Input: part model. Units: mm. Frame: model coordinates. A direction names the side the tool comes from. Give positions to 0.01 mm unless a question says otherwise; leave off trailing zeros. Order: outer loops, then holes, each group sorted by start corner. A loop starts at its lowest first (then second) coordinate and runs counter-clockwise, first axis right, second up. Notation, with made-up numbers: (68.25, 48.25) - (125.25, 48.25) arc R18 cw to (125.25, 67.25) - close; hole circle Ø2 at (-38.5, 8.25). An arc over 180 degrees is marked (long way). Answer in a Markdown table with one row per item. Add a question column.
1. Contact query for flat-ended pins moving along their axis: pin 1 (1.5 mm diameter, centred on y = 31.5, z = 6.5, fed in from +X); pin 2 (0.7 mm diameter, centred on y = 34.5, z = 516, fed in from +X); pin 3 (5 mm diameter, centred on x = -1, z = 219.5, fed in from +Y). Output: stop coordinate, or through.
2. Ray query, line 1 (Z direction, x = 4.5, y = 17.5); line 2 (Z direction, x = -6.5, y = 12); line 3 (Y direction, x = 6.25, z = 305). Return the intervals inside material, ascending. Write a range as [from, to].
3. Section query A-A on z = 353.5. Return loops of the section in (x, y), and give its area (3 significant figures).
4. Access query for faces 5 (the face through (-1, 15, 11)), 6 (the face through (7.5, 15.6, 521.3)), 7 (the face through (11.9, 16, 2)). Directions: +Z, -Z, +X, -X, +Y, -Y. A direction counts if a zero-diameter tool reaches every point of the face in a straight line with its end or side. Return the directions, or none.
5. Mould query, pull axis X, two halves, no side actions, for faces 1 (the face through (5, 34.5, 259)), 2 (the face through (-1, 16, 5)), 3 (the face through (-12.5, 15, 259)), 4 (the face through (7.5, 15.6, 4.7)). Classes: released by +X, released by -X, zero draft, split by the parting line, or undercut.
```python
from build123d import *

# Parameters (mm, degrees)
EXTRUDE_1_DEPTH          = 526
SKETCH_2_W               = 10
SKETCH_2_H               = 0.6
CUT_EXTRUDE_1_DEPTH      = 14.5
EXTRUDE_START            = -12.5
EXTRUDE_2_DEPTH          = 5
CUT_EXTRUDE_2_DEPTH      = 4.4
CUT_EXTRUDE_3_DEPTH      = 26
CUT_EXTRUDE_4_DEPTH      = 5.5
CUT_EXTRUDE_4_DEPTH_BACK = 5.5
CUT_EXTRUDE_5_DEPTH      = 35.5
SKETCH_8_W               = 0.5
SKETCH_8_H               = 1
CUT_EXTRUDE_8_DEPTH      = 491


with BuildPart() as part:
    # Эскиз1 → Бобышка-Вытянуть1 (new body)
    with BuildSketch(Plane.XY):
        with BuildLine():
            Line((-11.8, 32.5), (-11.8, 28.3))
            Line((-11.8, 28.3), (-11, 27.5))
            Line((-11, 27.5), (-11, 26))
            Line((-11, 26), (-12.5, 24.5))
            Line((-12.5, 24.5), (-12.5, 5))
            ThreePointArc((-12.5, 5), (-11.035533906, 1.464466094), (-7.5, 0))
            Line((-7.5, 0), (7.5, 0))
            ThreePointArc((7.5, 0), (11.035533906, 1.464466094), (12.5, 5))
            Line((12.5, 5), (12.5, 26.5))
            Line((12.5, 26.5), (11.7, 27.3))
            Line((11.7, 27.3), (11.7, 28.5))
            Line((11.7, 28.5), (12.5, 29.3))
            Line((12.5, 29.3), (12.5, 32.5))
            ThreePointArc((12.5, 32.5), (11.914213562, 33.914213562), (10.5, 34.5))
            Line((10.5, 34.5), (-9.8, 34.5))
            ThreePointArc((-9.8, 34.5), (-11.214213562, 33.914213562), (-11.8, 32.5))
        make_face()
    extrude(amount=EXTRUDE_1_DEPTH)

    # Эскиз2 → Вырез-Вытянуть1 (cut)
    with BuildSketch(Plane(origin=(0, 0, 0), x_dir=(-1, 0, 0), z_dir=(0, 0, -1))):
        with BuildLine():
            ThreePointArc((-10.5, 33.9), (-11.489949494, 33.489949494), (-11.9, 32.5))
            Line((-11.9, 32.5), (-11.9, 29.548528137))
            Line((-11.9, 29.548528137), (-11.1, 28.748528137))
            Line((-11.1, 28.748528137), (-11.1, 27.051471863))
            Line((-11.1, 27.051471863), (-11.9, 26.251471863))
            Line((-11.9, 26.251471863), (-11.9, 5))
            ThreePointArc((-11.9, 5), (-10.611269837, 1.888730163), (-7.5, 0.6))
            Line((-7.5, 0.6), (-7.5, 0))
            ThreePointArc((-7.5, 0), (-11.035533906, 1.464466094), (-12.5, 5))
            Line((-12.5, 5), (-12.5, 26.5))
            Line((-12.5, 26.5), (-11.7, 27.3))
            Line((-11.7, 27.3), (-11.7, 28.5))
            Line((-11.7, 28.5), (-12.5, 29.3))
            Line((-12.5, 29.3), (-12.5, 32.5))
            ThreePointArc((-12.5, 32.5), (-11.914213562, 33.914213562), (-10.5, 34.5))
            Line((-10.5, 34.5), (-10.5, 33.9))
        make_face()
        with Locations((0, 0.3)):
            Rectangle(SKETCH_2_W, SKETCH_2_H)
    cut_extrude_1 = extrude(amount=-CUT_EXTRUDE_1_DEPTH, mode=Mode.SUBTRACT)

    # Эскиз5 → Бобышка-Вытянуть2 (add)
    with BuildSketch(Plane.XY.offset(526).offset(EXTRUDE_START)):
        Polygon((-4.5, 34.5), (-2.7, 36.3), (2.7, 36.3), (4.5, 34.5), align=None)
    extrude_2 = extrude(amount=-EXTRUDE_2_DEPTH)

    # Зеркальное отражение1: Вырез-Вытянуть1, Бобышка-Вытянуть2 across plane
    add(cut_extrude_1.mirror(Plane.XY.offset(263)), mode=Mode.SUBTRACT)
    add(extrude_2.mirror(Plane.XY.offset(263)))

    # Эскиз3 → Вырез-Вытянуть2 (cut)
    with BuildSketch(Plane(origin=(11.9, 0, 0), x_dir=(0, 0, -1), z_dir=(1, 0, 0))):
        with BuildLine():
            Line((-523, 14), (-523, 17))
            ThreePointArc((-523, 17), (-518, 22), (-513, 17))
            Line((-513, 17), (-513, 14))
            ThreePointArc((-513, 14), (-518, 9), (-523, 14))
        make_face()
        with BuildLine():
            Line((-3, 14), (-3, 17))
            ThreePointArc((-3, 17), (-8, 22), (-13, 17))
            Line((-13, 17), (-13, 14))
            ThreePointArc((-13, 14), (-8, 9), (-3, 14))
        make_face()
    extrude(amount=-CUT_EXTRUDE_2_DEPTH, mode=Mode.SUBTRACT)

    # Эскиз4 → Вырез-Вытянуть3 (cut, through all)
    with BuildSketch(Plane(origin=(12.5, 0, 0), x_dir=(0, 0, -1), z_dir=(1, 0, 0))):
        with BuildLine():
            Line((-521, 14), (-521, 17))
            ThreePointArc((-521, 17), (-518, 20), (-515, 17))
            Line((-515, 17), (-515, 14))
            ThreePointArc((-515, 14), (-518, 11), (-521, 14))
        make_face()
        with BuildLine():
            Line((-5, 14), (-5, 17))
            ThreePointArc((-5, 17), (-8, 20), (-11, 17))
            Line((-11, 17), (-11, 14))
            ThreePointArc((-11, 14), (-8, 11), (-5, 14))
        make_face()
    extrude(amount=-CUT_EXTRUDE_3_DEPTH, mode=Mode.SUBTRACT)

    # Эскиз6 → Вырез-Вытянуть4 (cut, two sides)
    with BuildSketch(Plane(origin=(0, 34.5, 0), x_dir=(1, 0, 0), z_dir=(0, 1, 0))) as cut_extrude_4_sk:
        with BuildLine():
            Line((-1.5, -3), (1.5, -3))
            ThreePointArc((1.5, -3), (6.5, -8), (1.5, -13))
            Line((1.5, -13), (-1.5, -13))
            ThreePointArc((-1.5, -13), (-6.5, -8), (-1.5, -3))
        make_face()
        with BuildLine():
            Line((-1.5, -513), (1.5, -513))
            ThreePointArc((1.5, -513), (6.5, -518), (1.5, -523))
            Line((1.5, -523), (-1.5, -523))
            ThreePointArc((-1.5, -523), (-6.5, -518), (-1.5, -513))
        make_face()
    extrude(amount=CUT_EXTRUDE_4_DEPTH, mode=Mode.SUBTRACT)
    extrude(cut_extrude_4_sk.sketch, amount=-CUT_EXTRUDE_4_DEPTH_BACK, mode=Mode.SUBTRACT)

    # Эскиз7 → Вырез-Вытянуть5 (cut, through all)
    with BuildSketch(Plane(origin=(0, 34.5, 0), x_dir=(1, 0, 0), z_dir=(0, 1, 0))):
        with BuildLine():
            Line((-1.5, -515), (1.5, -515))
            ThreePointArc((1.5, -515), (4.5, -518), (1.5, -521))
            Line((1.5, -521), (-1.5, -521))
            ThreePointArc((-1.5, -521), (-4.5, -518), (-1.5, -515))
        make_face()
        with BuildLine():
            Line((-1.5, -5), (1.5, -5))
            ThreePointArc((1.5, -5), (4.5, -8), (1.5, -11))
            Line((1.5, -11), (-1.5, -11))
            ThreePointArc((-1.5, -11), (-4.5, -8), (-1.5, -5))
        make_face()
    extrude(amount=-CUT_EXTRUDE_5_DEPTH, mode=Mode.SUBTRACT)

    # Эскиз8 → Вырез-Вытянуть8 (cut)
    with BuildSketch(Plane.XY.offset(17.5)):
        Polygon((-0.25, 34.5), (-4.5, 34.5), (-4.5, 33.5), align=None)
        with Locations((0, 34)):
            Rectangle(SKETCH_8_W, SKETCH_8_H)
        Polygon((4.5, 34.5), (0.25, 34.5), (4.5, 33.5), align=None)
    extrude(amount=CUT_EXTRUDE_8_DEPTH, mode=Mode.SUBTRACT)


solid = part.part
```
Answer:
| question | item | result |
|---|---|---|
| 1 | pin 1 | stops at x = 11.9 |
| 1 | pin 2 | stops at x = 10.5 |
| 1 | pin 3 | stops at y = 34.5 |
| 2 | line 1 | z = [0, 5.04], [10.96, 515.04], [520.96, 526] |
| 2 | line 2 | z = [0, 5.76], [10.24, 515.76], [520.24, 526] |
| 2 | line 3 | y = [0, 34.5] |
| 3 | outline | (-12.5, 5) arc R5 ccw to (-7.5, 0) - (7.5, 0) arc R5 ccw to (12.5, 5) - (12.5, 26.5) - (11.7, 27.3) - (11.7, 28.5) - (12.5, 29.3) - (12.5, 32.5) arc R2 ccw to (10.5, 34.5) - (4.5, 34.5) - (4.5, 33.5) - (0.25, 34.5) - (0.25, 33.5) - (-0.25, 33.5) - (-0.25, 34.5) - (-4.5, 33.5) - (-4.5, 34.5) - (-9.8, 34.5) arc R2 ccw to (-11.8, 32.5) - (-11.8, 28.3) - (-11, 27.5) - (-11, 26) - (-12.5, 24.5) - close |
| 3 | area | 835 mm² |
| 4 | face 5 | none |
| 4 | face 6 | +X |
| 4 | face 7 | -Z, +X, +Y, -Y |
| 5 | face 1 | zero draft |
| 5 | face 2 | undercut |
| 5 | face 3 | released by -X |
| 5 | face 4 | released by +X |
